Drawing for the job (mm, zero at the part's lowest x, y, z). A direction names the side the tool comes from. Round coordinates to 2 decimals unless told otherwise and drop trailing zeros. Order: outer loops, then holes, each group sorted by start corner. A loop starts at its lowest first (then second) coordinate and runs counter-clockwise, first axis right, second up. Notation, with made-up numbers: M 64,-24.5 L 100,-24.5 A18 cw 100,-11.5 Z; hole C 35.5,44 d7. An arc over 180 degrees is marked long. Answer as CSV lines item,"result". Start each with the question number.
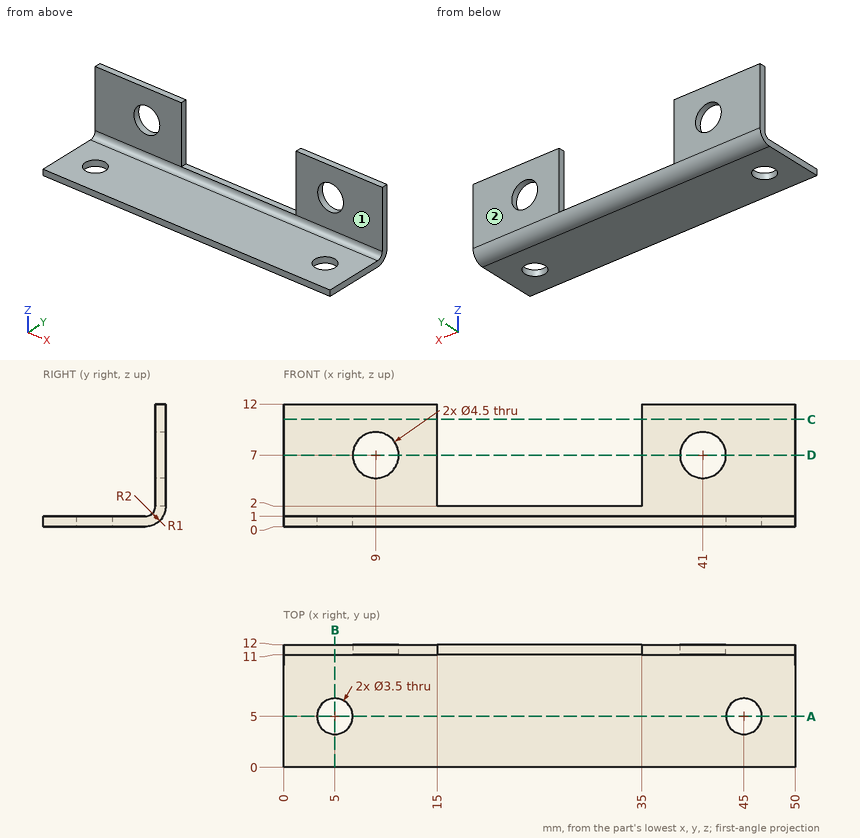
Q1. Band-saw the part on B-B, the plane x = 5. Write the cut outline in (y, z).
Q2. Tool access for the marked faces 1 and 2: list every direction of +Z, -Z, +X, -X, +Y, -Y with a clear straight run to the whole face (end or side of a thin tool).
Q3. Band-saw the part on D-D, the plane z = 7. Write the cut outline in (x, y), then the cut area to 3 significant figures.
Q4. Band-saw the part on C-C, the plane z = 10.5. Write the cut outline in (x, y).
Q5. Drop flat-ended pins along their axis: P1, Ø3, axis at x = 36.5, y = 5.5, coming from the +Z side; P2, Ø3, axis at y = 9, z = 1.5, coming from the -X side; P3, Ø1.5, axis at y = 10, z = 4.5, coming from the -X side; P4, Ø0.5, axis at x = 26, y = 11.5, coming from the +Z side. Give the stop position or say it passes through.
Q6. Probe line 1 along Z through (x, y) = (44, 8); line 2 along Y through (x, z) = (5, 0.8); line 3 along Y through (x, z) = (6, 9.75). List the from-to ranges inside material, lowest first. Write a range as from..to.
Q7. Band-saw the part on A-A, the plane y = 5. Write the cut outline in (x, z).
Answer:
1,outline,"M 0,0 L 3.25,0 L 3.25,1 L 0,1 Z; M 6.75,0 L 10,0 A2 ccw 12,2 L 12,12 L 11,12 L 11,2 A1 cw 10,1 L 6.75,1 Z"
2,face 1,"+Z, +X, -X, -Y"
2,face 2,"+Z, -Z, +X, -X, +Y"
3,outline,"M 0,11 L 6.75,11 L 6.75,12 L 0,12 Z; M 11.25,11 L 15,11 L 15,12 L 11.25,12 Z; M 35,11 L 38.75,11 L 38.75,12 L 35,12 Z; M 43.25,11 L 50,11 L 50,12 L 43.25,12 Z"
3,area,"21.0 mm^2"
4,outline,"M 0,11 L 15,11 L 15,12 L 0,12 Z; M 35,11 L 50,11 L 50,12 L 35,12 Z"
5,P1,"stops at z = 1"
5,P2,"stops at x = 0"
5,P3,"passes through"
5,P4,"stops at z = 2"
6,line 1,"z = 0..1"
6,line 2,"y = 0..3.25, 6.75..11.6"
6,line 3,"y = 11..12"
7,outline,"M 0,0 L 3.25,0 L 3.25,1 L 0,1 Z; M 6.75,0 L 43.25,0 L 43.25,1 L 6.75,1 Z; M 46.75,0 L 50,0 L 50,1 L 46.75,1 Z"
